Design review of the part built by this model. Coordinates are the model's own, in mm. A direction names the side the tool comes from. Round coordinates to 2 decimals unless told otherwise and drop trailing zeros. Loops run counter-clockwise (first coordinate to the right, second up) from the corner with the lowest first, then second, coordinate; pieces in that order, holes last. Notation, with made-up numbers: M -29.5,53.25 L -10.5,53.25 A22 cw -10.5,73.25 Z; hole C 79.5,-11.75 d11. An arc over 180 degrees is marked long. One line per item, written item: value. Start each with the question number.
Item 1: We need section C-C (y = -54). Write out the cut boundary in (x, z) (3 decimals), then the cut area to 3 significant figures.
Item 2: We need section D-D (x = 85). Write out the cut boundary in (y, z) (3 decimals).
Item 3: We need section B-B (x = 65.5). Write out the cut boundary in (y, z) (3 decimals), then the cut area to 3 significant figures.
Item 4: Clearance check with flat-ended pins moving along their axes: pin 1 (6 mm diameter, centred on x = 69.5, z = 44.5, fed in from -Y); pin 2 (5 mm diameter, centred on y = 1.5, z = 46.5, fed in from -X); pin 3 (12 mm diameter, centred on y = 3.5, z = 17, fed in from +X) (3 decimals). State where each tip first meets the part, or that it passes through.
Item 5: Mouldability with a two-part tool opening along X and no side actions: class faces 5 (the flat face through (59, 4, 42.875)), 6 (the flat face through (22.225, -17, 18)), 7 (the flat face through (59.6, -2, 61.925)) as released by +X, released by -X, zero draft, split by the parting line, or undercut.
Item 6: For faces 1 (the cylindrical face through (39.46, -41.5, 7.62)), 2 (the flat face through (41.275, 12, 8)), 3 (the cylindrical face through (30.59, 16.55, 49.68)), 4 (the flat face through (6, -7.938, 30)), list the 3-axis set-ups (+Z, -Z, +X, -X, +Y, -Y) from which the entire face can be reached by the end or side of a thin tool; tool diameter is ignored.
Item 7: For line 1 along Y through (x, z) = (5, 21); line 2 along Y through (x, z) = (27, 19.5); line 3 along Z through (x, y) = (11, 54.5) (3 decimals), list the stretches that pass through material, from the lowest coordinate up.
Item 8: We need section A-A (y = 42). Write out the cut boundary in (x, z) (3 decimals), then the cut area to 3 significant figures.
from build123d import *

# Parameters (mm, degrees)
F1_DEPTH = 63.5
F2_DEPTH = 7.9375
F0_W     = 25.2498040683
F0_H     = 19.05
F3_DEPTH = 25.4
F5_R     = 6.35


# Not quite as in the source:
# - a feature names something its author has since deleted; it is built from what else it names


with BuildPart() as f1:
    # F0 (on Front) → F1 (new body, symmetric)
    with BuildSketch(Plane.XZ):
        Polygon((-41.275, -9.525), (41.275, -9.525), (41.275, 9.525), (22.225, 9.525), (-41.275, 9.525), align=None)
    extrude(amount=F1_DEPTH, both=True)

    # F0 (on Front) → F2 (join, symmetric)
    with BuildSketch(Plane.XZ):
        with BuildLine():
            add(Edge.make_bspline(
                [(-41.275, 9.525), (-23.4670489943, 36.4343195367), (10.3939996221, 56.9389145817), (51.0054120889, 61.3804219947)],
                knots=[0, 0, 0, 0, 106.1920094682, 106.1920094682, 106.1920094682, 106.1920094682], degree=3))
            Line((-41.275, 9.525), (22.225, 9.525))
            Line((22.225, 9.525), (22.225, 27.0002))
            ThreePointArc((22.225, 27.0002), (30.3698267575, 49.4184502908), (51.0054120889, 61.3804219947))
        make_face()
    extrude(amount=F2_DEPTH, both=True)

    # F0 (on Front) → F3 (join, symmetric)
    with BuildSketch(Plane.XZ):
        with BuildLine():
            Line((22.225, 9.525), (41.275, 9.525))
            Line((41.275, 9.525), (41.275, 27.0002))
            ThreePointArc((41.275, 27.0002), (45.9246798487, 38.2255201513), (57.15, 42.8752))
            Line((57.15, 42.8752), (60.325, 42.8752))
            Line((60.325, 42.8752), (60.325, 61.9252))
            Line((60.325, 61.9252), (57.15, 61.9252))
            add(Edge.make_bspline(
                [(51.0054120889, 61.3804219947), (53.0371017984, 61.6026197553), (55.0856860239, 61.7846155213), (57.15, 61.9252)],
                knots=[106.1920094682, 106.1920094682, 106.1920094682, 106.1920094682, 111.5045361635, 111.5045361635, 111.5045361635, 111.5045361635], degree=3))
            ThreePointArc((51.0054120889, 61.3804219947), (30.3698267575, 49.4184502908), (22.225, 27.0002))
            Line((22.225, 27.0002), (22.225, 9.525))
        make_face()
        with Locations((72.9499020342, 52.4002)):
            Rectangle(F0_W, F0_H)
    extrude(amount=F3_DEPTH, both=True)

    # F0 (on Front) → F4 (revolve)
    with BuildSketch(Plane.XZ):
        Polygon((85.5748040683, 61.9252), (85.5748040683, 42.8752), (85.5748040683, 38.1), (111.125, 38.1), (111.125, 66.675), (85.5748040683, 66.675), align=None)
    revolve(axis=Axis((85.5748040683, 0, 52.3875), (0, 0, -1)))

    # F5
    f5_edges = [f1.edges().sort_by_distance(p)[0] for p in [
        (41.275, -63.5, 0),
        (-41.275, -63.5, 0),
        (0, -63.5, 9.525),
        (41.275, 0, -9.525),
        (0, -63.5, -9.525),
        (41.275, -44.45, 9.525),
        (-41.275, 63.5, 0),
        (41.275, 63.5, 0),
    ]]
    fillet(f5_edges, radius=F5_R)


solid = f1.part
A:
1. outline: M -41.275,-9.525 L 34.925,-9.525 A6.35 ccw 41.275,-3.175 L 41.275,3.175 A6.35 ccw 34.925,9.525 L -41.275,9.525 Z
1. area: 1,560 mm2
2. outline: M -25.544,38.1 L 25.544,38.1 L 25.544,66.675 L -25.544,66.675 Z
3. outline: M -25.4,42.875 L -15.806,42.875 L -15.806,38.1 L 15.806,38.1 L 15.806,42.875 L 25.4,42.875 L 25.4,61.925 L 15.806,61.925 L 15.806,66.675 L -15.806,66.675 L -15.806,61.925 L -25.4,61.925 Z
3. area: 1,270 mm2
4. pin 1: y = -25.4
4. pin 2: x = -3.47
4. pin 3: x = 41.275
5. face 5: undercut
5. face 6: released by -X
5. face 7: zero draft
6. face 1: +Z, +X, -Y
6. face 2: -Z, +X, +Y, -Y
6. face 3: +Z, -X, +Y
6. face 4: +Z, -X, -Y
7. line 1: -7.94 to 7.94
7. line 2: -25.4 to 25.4
7. line 3: -9.525 to 9.525
8. outline: M -41.275,-9.525 L 34.925,-9.525 A6.35 ccw 41.275,-3.175 L 41.275,9.525 L -41.275,9.525 Z
8. area: 1,560 mm2
